Answer from the drawing. Dimensions are ordinates in mm from the lowest x, y and z of the part. A direction names the side the tool comes from. Round coordinates to 2 decimals unless told otherwise and drop trailing zeros. Write each loop counter-clockwise with the first axis right and the second up, starting at its lowest first coordinate (ties: lowest second). Pieces come first, ordered by that corner, then holes. Notation, with made-up numbers: (36.25, 69) - (75.25, 69) arc R16 cw to (75.25, 90) - close; hole circle Ø2 at (82.5, 25). An arc over 180 degrees is marked (long way). Answer as CSV lines item,"result". Start each with the question number.
1) Consider line 1 along Z through (x, y) = (11, 8); line 2 along X through (y, z) = (8, 3.5). Determine where each line is inside the solid, lowest interval first.
2) Which of the six approach directions +Z, -Z, +X, -X, +Y, -Y give full straight-line access (tool end or side, diameter ignored) to the marked faces 4 and 5?
3) For a pull along Z with two mould halves and no side action, classify the marked faces 1, 2 and 3 as +Z half, -Z half, draft (parallel to the pull), parting line (faces both ways), or undercut.
4) Find section A-A on x = 14.25. Determine the outline of the cut face in (y, z).
5) Find section B-B on y = 1.5. Determine the outline of the cut face in (x, z), then the cut area to 3 significant figures.
6) Each of these flat-tipped pins is pushed along its axis until it touches: pin 1 (0.6 mm diameter, centred on y = 3, z = 3.5, fed in from -X); pin 2 (2 mm diameter, centred on x = 7, y = 6, fed in from -Z); pin 3 (0.7 mm diameter, centred on y = 3.5, z = 4, fed in from +X); pin 4 (0.8 mm diameter, centred on y = 2.5, z = 4.5, fed in from -X). Where does it stop, or does it pass through?
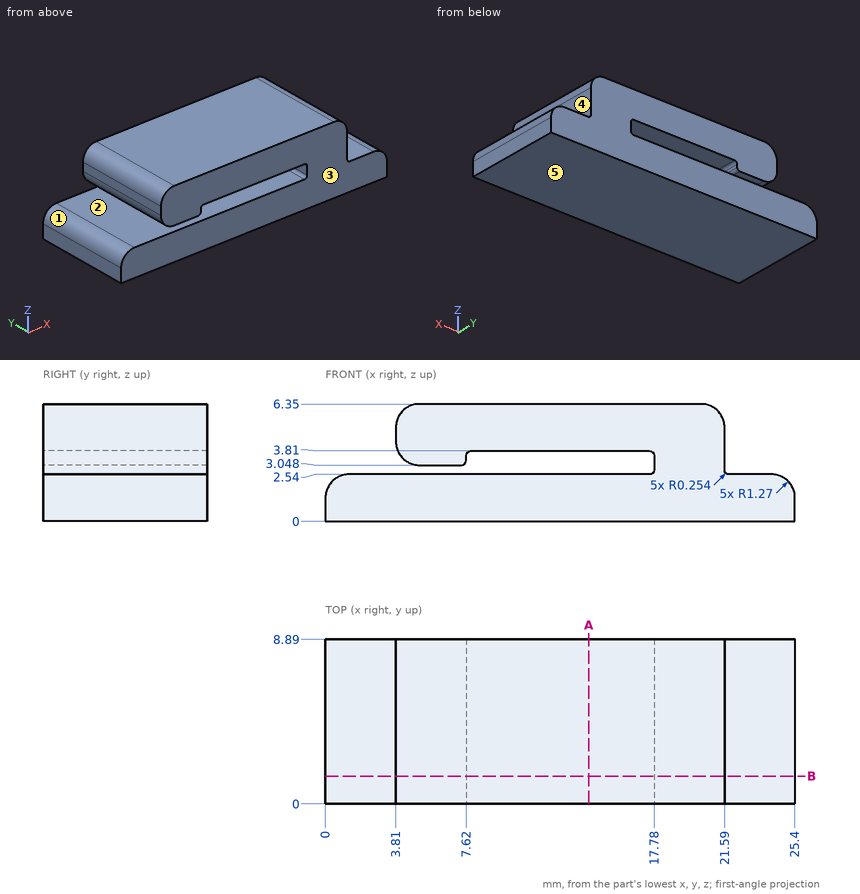
Check values:
1,line 1,"z = 0 to 2.54, 3.81 to 6.35"
1,line 2,"x = 4.11 to 7.62, 17.78 to 21.59"
2,face 4,"+Z, +X, +Y, -Y"
2,face 5,"-Z, +X, -X, +Y, -Y"
3,face 1,"+Z half"
3,face 2,"undercut"
3,face 3,"draft"
4,outline,"(0, 0) - (8.89, 0) - (8.89, 2.54) - (0, 2.54) - close; (0, 3.81) - (8.89, 3.81) - (8.89, 6.35) - (0, 6.35) - close"
5,outline,"(0, 0) - (25.4, 0) - (25.4, 1.27) arc R1.27 ccw to (24.13, 2.54) - (21.84, 2.54) arc R0.25 cw to (21.59, 2.79) - (21.59, 5.08) arc R1.27 ccw to (20.32, 6.35) - (5.08, 6.35) arc R1.27 ccw to (3.81, 5.08) - (3.81, 4.32) arc R1.27 ccw to (5.08, 3.05) - (7.37, 3.05) arc R0.25 ccw to (7.62, 3.3) - (7.62, 3.56) arc R0.25 cw to (7.87, 3.81) - (17.53, 3.81) arc R0.25 cw to (17.78, 3.56) - (17.78, 2.79) arc R0.25 cw to (17.53, 2.54) - (1.27, 2.54) arc R1.27 ccw to (0, 1.27) - close"
5,area,"116 mm^2"
6,pin 1,"stops at x = 3.92"
6,pin 2,"stops at z = 0"
6,pin 3,"stops at x = 21.59"
6,pin 4,"stops at x = 3.81"
